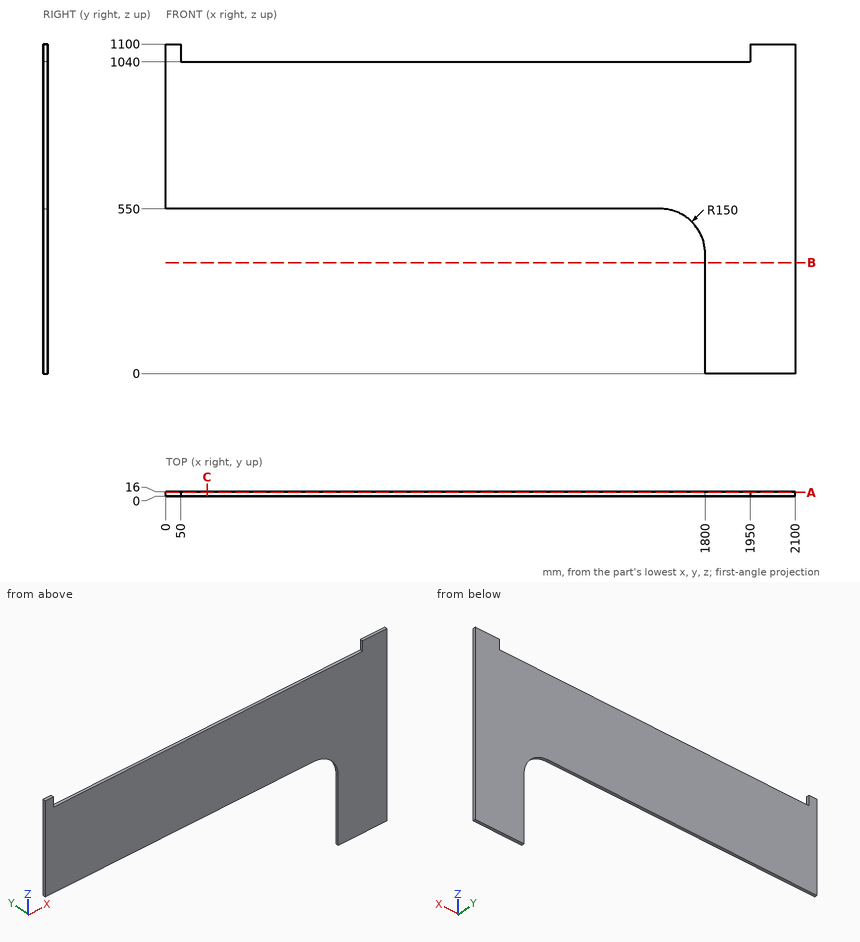
Could you check a few things on this drawing? It's one solid part, dimensions in mm from its lowest x, y, z. Coordinates: 2 decimals unless noted, no trailing zeros. Order: outer loops, then holes, each group sorted by start corner. A loop starts at its lowest first (then second) coordinate and runs counter-clockwise, first axis right, second up.
1. I need wall thicknesses on line 1 (X direction, y = 8.25, z = 303.5); line 2 (Z direction, x = 462.5, y = 5.75); line 3 (Z direction, x = 1870, y = 8.75). Which ranges of each line are inside material? Lowest first, please.
2. If we section it at C-C (x = 138): Please give me the cut outline in (y, z).
3. If we section it at B-B (z = 370): Please give me the cut outline in (x, y), then the cut area to 3 significant figures.
4. I'm going to push flat-ended pins straight in: pin 1 (8 mm diameter, centred on x = 460.5, y = 8, fed in from -Z); pin 2 (2 mm diameter, centred on y = 9, z = 240, fed in from -X); pin 3 (8 mm diameter, centred on x = 1439.5, y = 8.5, fed in from +Z). Where does each tip first touch, or does it pass through?
5. If we section it at A-A (y = 13): Please give me the cut outline in (x, z).
Entries:
1. line 1: x = 1800 to 2100
1. line 2: z = 550 to 1040
1. line 3: z = 0 to 1040
2. outline: (0, 550) - (16, 550) - (16, 1040) - (0, 1040) - close
3. outline: (1800, 0) - (2100, 0) - (2100, 16) - (1800, 16) - close
3. area: 4,800 mm2
4. pin 1: stops at z = 550
4. pin 2: stops at x = 1800
4. pin 3: stops at z = 1040
5. outline: (0, 550) - (1650, 550) arc R150 cw to (1800, 400) - (1800, 0) - (2100, 0) - (2100, 1100) - (1950, 1100) - (1950, 1040) - (50, 1040) - (50, 1100) - (0, 1100) - close
